Model file for the job. Use its own axes, mm. Round coordinates to 2 decimals unless told otherwise and drop trailing zeros. Order: outer loops, then holes, each group sorted by start corner. A loop starts at its lowest first (then second) coordinate and runs counter-clockwise, first axis right, second up. Notation, with made-up numbers: (43.5, 79.5) - (62.5, 79.5) arc R19 cw to (62.5, 103.5) - close; hole circle Ø8 at (66, 75.25). An arc over 180 degrees is marked (long way). Put each result on its own line as item: value. Start each with the question number.
Item 1: Probe probe 1 along X at (y, z) = (30, 0.85); probe 2 along X at (y, z) = (31.5, 1.2); probe 3 along X at (y, z) = (-1, 0.55). List the from-to ranges inside material, lowest first.
Item 2: Saw through at C-C on z = 1.4. State how many separate pieces and enclosed holes the cut face has, plus the area to 3 significant figures.
Item 3: Pin check, flat tips, straight feed: pin 1 Ø2 at (x, y) = (8.13, 8.13) entering from +Z; pin 2 Ø1 at (y, z) = (21, 1) entering from -X; pin 3 Ø1.5 at (x, y) = (-36.5, 11) entering from -Z; pin 4 Ø1 at (x, z) = (-29.5, 0.5) entering from -Y. Stop position of each tip, or through.
Item 4: Saw through at A-A on x = 11.5. List the corners of the cut face in (y, z).
Item 5: Saw through at B-B on x = -23.5. List the corners of the cut face in (y, z).
Item 6: Saw through at D-D on x = -12. List the corners of the cut face in (y, z).
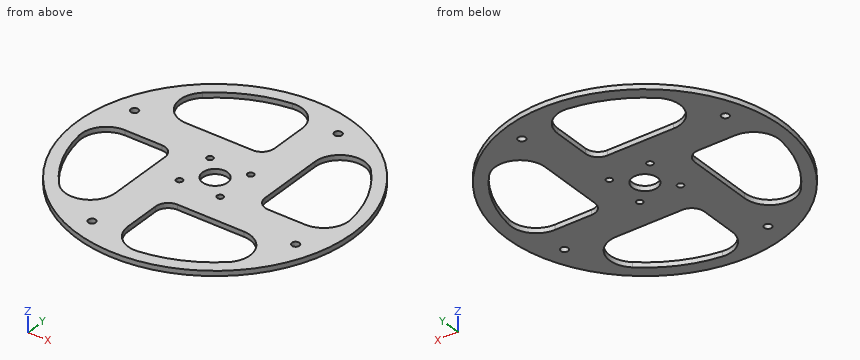
```python
from build123d import *

# Parameters (mm, degrees)
SKETCH_1_R      = 55
SKETCH_1_R_2    = 1.5
SKETCH_1_R_3    = 1.25
SKETCH_1_R_4    = 5
EXTRUDE_1_DEPTH = 2


with BuildPart() as part:
    # 草图1 → 凸台-拉伸1 (new body)
    with BuildSketch(Plane.XY):
        Circle(SKETCH_1_R)
        with Locations((-16.074946736, -44.165553177)):
            Circle(SKETCH_1_R_2, mode=Mode.SUBTRACT)
        with BuildLine():
            Line((-39.686269666, 5), (-25, 5))
            ThreePointArc((-25, 5), (-21.464466094, 3.535533906), (-20, 0))
            Line((-20, 0), (-20, -26.457513111))
            ThreePointArc((-20, -26.457513111), (-26.464466094, -35.811656578), (-37.5, -33.071891388))
            ThreePointArc((-37.5, -33.071891388), (-45.571891388, -20.571891388), (-49.607837082, -6.25))
            ThreePointArc((-49.607837082, -6.25), (-47.186269666, 1.614378278), (-39.686269666, 5))
        make_face(mode=Mode.SUBTRACT)
        with Locations((-8.131727984, -8.131727984)):
            Circle(SKETCH_1_R_3, mode=Mode.SUBTRACT)
        with BuildLine():
            ThreePointArc((-5, -25), (-3.535533906, -21.464466094), (0, -20))
            Line((0, -20), (26.457513111, -20))
            ThreePointArc((26.457513111, -20), (35.811656578, -26.464466094), (33.071891388, -37.5))
            ThreePointArc((33.071891388, -37.5), (20.571891388, -45.571891388), (6.25, -49.607837082))
            ThreePointArc((6.25, -49.607837082), (-1.614378278, -47.186269666), (-5, -39.686269666))
            Line((-5, -39.686269666), (-5, -25))
        make_face(mode=Mode.SUBTRACT)
        with Locations((8.131727984, -8.131727984)):
            Circle(SKETCH_1_R_3, mode=Mode.SUBTRACT)
        with Locations((44.165553177, -16.074946736)):
            Circle(SKETCH_1_R_2, mode=Mode.SUBTRACT)
        with Locations((-44.165553177, 16.074946736)):
            Circle(SKETCH_1_R_2, mode=Mode.SUBTRACT)
        with Locations((-8.131727984, 8.131727984)):
            Circle(SKETCH_1_R_3, mode=Mode.SUBTRACT)
        with BuildLine():
            ThreePointArc((5, 25), (3.535533906, 21.464466094), (0, 20))
            Line((0, 20), (-26.457513111, 20))
            ThreePointArc((-26.457513111, 20), (-35.811656578, 26.464466094), (-33.071891388, 37.5))
            ThreePointArc((-33.071891388, 37.5), (-20.571891388, 45.571891388), (-6.25, 49.607837082))
            ThreePointArc((-6.25, 49.607837082), (1.614378278, 47.186269666), (5, 39.686269666))
            Line((5, 39.686269666), (5, 25))
        make_face(mode=Mode.SUBTRACT)
        Circle(SKETCH_1_R_4, mode=Mode.SUBTRACT)
        with Locations((8.131727984, 8.131727984)):
            Circle(SKETCH_1_R_3, mode=Mode.SUBTRACT)
        with BuildLine():
            ThreePointArc((25, -5), (21.464466094, -3.535533906), (20, 0))
            Line((20, 0), (20, 26.457513111))
            ThreePointArc((20, 26.457513111), (26.464466094, 35.811656578), (37.5, 33.071891388))
            ThreePointArc((37.5, 33.071891388), (45.571891388, 20.571891388), (49.607837082, 6.25))
            ThreePointArc((49.607837082, 6.25), (47.186269666, -1.614378278), (39.686269666, -5))
            Line((39.686269666, -5), (25, -5))
        make_face(mode=Mode.SUBTRACT)
        with Locations((16.074946736, 44.165553177)):
            Circle(SKETCH_1_R_2, mode=Mode.SUBTRACT)
    extrude(amount=EXTRUDE_1_DEPTH)


solid = part.part
```
Results found:
1. probe 1: x = -46.1 to -36.46, 5 to 20.65, 40 to 46.1
1. probe 2: x = -45.09 to -36.34, 5 to 21.36, 38.83 to 45.09
1. probe 3: x = -54.99 to -48.85, -20 to -4.9, 4.9 to 20.1, 47.69 to 54.99
2. separate pieces: 1
2. enclosed holes: 13
2. area: 5,330 mm²
3. pin 1: passes through
3. pin 2: stops at x = -51.04
3. pin 3: stops at z = 0
3. pin 4: stops at y = -46.73
4. outline: (-53.78, 0) - (-48.66, 0) - (-48.66, 2) - (-53.78, 2) - close; (-20, 0) - (53.78, 0) - (53.78, 2) - (-20, 2) - close
5. outline: (-49.73, 0) - (-34.06, 0) - (-34.06, 2) - (-49.73, 2) - close; (4.77, 0) - (20, 0) - (20, 2) - (4.77, 2) - close; (44.13, 0) - (49.73, 0) - (49.73, 2) - (44.13, 2) - close
6. outline: (-53.67, 0) - (20, 0) - (20, 2) - (-53.67, 2) - close; (48.54, 0) - (53.67, 0) - (53.67, 2) - (48.54, 2) - close
